```python
from build123d import *

# Parameters (mm, degrees)
F1_DEPTH      = 140
F1_TAPER      = 7
F1_DEPTH_BACK = 50
F1_TAPER_BACK = 18
F3_DEPTH      = 2
F4_R          = 12
F5_DEPTH      = 50


with BuildPart() as f1:
    # F0 (on Front) → F1 (new body, two sides)
    with BuildSketch(Plane.XZ) as f1_sk:
        Polygon((0, 20), (-40, 0), (0, -20), (40, 0), align=None)
    extrude(amount=F1_DEPTH, taper=F1_TAPER)
    extrude(f1_sk.sketch, amount=-F1_DEPTH_BACK, taper=F1_TAPER_BACK)

    # F2 (on Top) → F3 (join, symmetric)
    with BuildSketch(Plane.XY):
        Polygon((0, 50), (0, -35), (75.0196278095, 30), (75.0196278095, 50), align=None)
        Polygon((-75.0196278095, 30), (0, -35), (0, 50), (-75.0196278095, 50), align=None)
    extrude(amount=F3_DEPTH, both=True)

    # F4 (on Front) → F5 (join)
    with BuildSketch(Plane.XZ):
        with BuildLine():
            ThreePointArc((0, 0), (12, -12), (24, 0))
            ThreePointArc((24, 0), (12, 12), (0, 0))
        make_face()
        with Locations((-12, 0)):
            Circle(F4_R)
    extrude(amount=-F5_DEPTH)


solid = f1.part
```
Here's how the part is built. I have some questions about the finished solid (model axes, mm). A direction names the side the tool comes from. Coordinates: 2 decimals unless noted, no trailing zeros. Order: outer loops, then holes, each group sorted by start corner. A loop starts at its lowest first (then second) coordinate and runs counter-clockwise, first axis right, second up.
1) I need wall thicknesses on line 1 (X direction, y = 30, z = -10); line 2 (Z direction, x = 67, y = 28); line 3 (Z direction, x = -18, y = -39). Which ranges of each line are inside material? Lowest first, please.
2) Imagine slicing it at A-A on x = -60. List the corners of the cut face in (y, z) for me.
3) Which directions (+Z, -Z, +X, -X, +Y, -Y) give clear straight access to the entire face, cutting with the end or side of a thin tool? Please do faces 1 (the face through (15.46, 30.84, -11.49)), 2 (the face through (-15.46, 30.84, 11.49)), 3 (the face through (49, 29, 2)).
4) Imagine slicing it at B-B on x = 52.5. List the corners of the cut face in (y, z) for me.
5) Will these pins go through, and if not, where does the flat tip stop? pin 1 (1 mm diameter, centred on x = 21, y = 16, fed in from -Z); pin 2 (6 mm diameter, centred on x = 24, y = 15, fed in from +Z); pin 3 (1 mm diameter, centred on y = -13.5, z = -9, fed in from -X); pin 4 (3 mm diameter, centred on x = 22, z = 12.5, fed in from -Y).
Response values:
1. line 1: x = -18.63 to -5.37, 5.37 to 18.63
1. line 2: z = -2 to 2
1. line 3: z = -5.65 to 5.65
2. outline: (16.99, -2) - (50, -2) - (50, 2) - (16.99, 2) - close
3. face 1: -Z, +Y
3. face 2: +Z, +Y
3. face 3: +Z, +X, +Y
4. outline: (10.49, -2) - (50, -2) - (50, 2) - (10.49, 2) - close
5. pin 1: stops at z = -8.47
5. pin 2: stops at z = 7.94
5. pin 3: stops at x = -19.3
5. pin 4: passes through
